from build123d import *

# Parameters (mm, degrees)
SKETCH008_W   = 384.79573
SKETCH008_H   = 385.031417
SKETCH008_W_2 = 376.917694
SKETCH008_H_2 = 377.136078
PAD007_DEPTH  = 38
SKETCH007_W   = 32
SKETCH007_H   = 377
PAD006_DEPTH  = 34
SKETCH009_W   = 384.911911
SKETCH009_H   = 384.509689
SKETCH009_W_2 = 310.483261
SKETCH009_H_2 = 308.455338
PAD008_DEPTH  = 4


with BuildPart() as body009:
    # Sketch008 (on Face1 of CopyClone001) → Pad007 (new body)
    with BuildSketch(Plane(origin=(135, 0, -118), x_dir=(1, 0, 0), z_dir=(0, 0, -1))):
        with Locations((-134.968895, 0.104423)):
            Rectangle(SKETCH008_W, SKETCH008_H)
        with Locations((-135.014908, -0.01149)):
            Rectangle(SKETCH008_W_2, SKETCH008_H_2, mode=Mode.SUBTRACT)
    extrude(amount=-PAD007_DEPTH)


with BuildPart() as body07:
    # Sketch007 (on Face1 of CopyPad005) → Pad006 (new body)
    with BuildSketch(Plane(origin=(0, 0, -84), x_dir=(1, 0, 0), z_dir=(0, 0, -1))):
        with Locations((-66.550887, -0.158425)):
            Rectangle(SKETCH007_W, SKETCH007_H)
    extrude(amount=PAD006_DEPTH)


with BuildPart() as body008:
    # Body008 base: copy of body07
    add(body07.part)


with BuildPart() as body008_1:
    # Clone001 placement: moved
    add(body008.part.moved(Location((135, 0, 0))))


with BuildPart() as baseplate:
    # Sketch009 (on Face1 of CopyPad006) → Pad008 (new body)
    with BuildSketch(Plane(origin=(0, 0, -118), x_dir=(1, 0, 0), z_dir=(0, 0, -1))):
        with Locations((0.316445, 0.346092)):
            Rectangle(SKETCH009_W, SKETCH009_H)
        with Locations((0.063926, 0.16024)):
            Rectangle(SKETCH009_W_2, SKETCH009_H_2, mode=Mode.SUBTRACT)
    extrude(amount=PAD008_DEPTH)

    # Boolean001: union Body009, Body008, body07
    add(body009.part)
    add(body008_1.part)
    add(body07.part)


solid = baseplate.part
Check sheet for the modelled part. Datum: model origin and axes. Units: mm. A direction names the side the tool comes from. Round coordinates to 2 decimals unless told otherwise and drop trailing zeros. Order: outer loops, then holes, each group sorted by start corner. A loop starts at its lowest first (then second) coordinate and runs counter-clockwise, first axis right, second up.
Q1. Set-up check for faces 1 (the face through (-192.367, 3, -99)), 2 (the face through (0, 171, -118)), 3 (the face through (-67, -2, -118)): record each of +Z, -Z, +X, -X, +Y, -Y from which the full face is reachable in a straight line by a thin tool's end or side.
Filled sheet:
face 1: +Z, -Z, -X, +Y, -Y
face 2: +Z
face 3: -Z
Q2. Depth check by flat-ended pin: P1, Ø4, axis at x = 57.5, y = 107.5, coming from the +Z side; P2, Ø19, axis at y = 83.5, z = -94.5, coming from the +X side; P3, Ø4.5, axis at x = -61, z = -120.5, coming from the +Y side; P4, Ø3, axis at y = -43, z = -119, coming from the -X side. Enter the tip coordinate at first touch or a pass-through.
Filled sheet:
P1: stops at z = -84
P2: stops at x = 192.43
P3: stops at y = 191.91
P4: stops at x = -192.37
Q3. Draft check along X on faces 4 (the face through (68, -2, -118)), 5 (the face through (192.429, 3, -99)), 6 (the face through (-3, 192.411, -99)), 7 (the face through (52.449, 3, -101)). Enter one of: pulls with the +X half, pulls with the -X half, needs draft (parallel to the pull), parting line crosses it, or undercut.
Filled sheet:
face 4: undercut
face 5: pulls with the +X half
face 6: needs draft
face 7: undercut
Q4. Scan lines: L1, parallel to X at y = 151, z = -87; L2, parallel to Y at x = 47.5, z = -98; L3, parallel to Y at x = -73, z = -97. Record each from-to range of solid material in increasing order.
Filled sheet:
L1: x = -192.37 to -188.47, -82.55 to -50.55, 52.45 to 84.45, 188.44 to 192.43
L2: y = -192.62 to -188.56, 188.58 to 192.41
L3: y = -192.62 to -188.56, -188.34 to 192.41
Q5. Cross-section at A-A, the plane y = -79. Enter the section's corners in (x, z).
Filled sheet:
outline: (-192.37, -118) - (-192.14, -118) - (-192.14, -122) - (-155.18, -122) - (-155.18, -118) - (-188.47, -118) - (-188.47, -80) - (-192.37, -80) - close; (-82.55, -118) - (-50.55, -118) - (-50.55, -84) - (-82.55, -84) - close; (52.45, -118) - (84.45, -118) - (84.45, -84) - (52.45, -84) - close; (155.31, -122) - (192.77, -122) - (192.77, -118) - (192.43, -118) - (192.43, -80) - (188.44, -80) - (188.44, -118) - (155.31, -118) - close
Q6. Cross-section at C-C, the plane z = -113. Enter the section's corners in (x, y).
Filled sheet:
outline: (-192.37, -192.62) - (192.43, -192.62) - (192.43, 192.41) - (-192.37, 192.41) - close; hole (-188.47, -188.56) - (188.44, -188.56) - (188.44, 188.58) - (84.45, 188.58) - (84.45, -188.34) - (52.45, -188.34) - (52.45, 188.58) - (-50.55, 188.58) - (-50.55, -188.34) - (-82.55, -188.34) - (-82.55, 188.58) - (-188.47, 188.58) - close
